Solid Edge part; units mm, degrees
sketch "Sketch1" plane through (0, 0, 0) normal (0, -1, 0) x (1, 0, 0)
  line L0 (0, -16) -> (1.5, -16)
  line L1 (1.5, -16) -> (1.5, -0.601)
  line L2 (1.5, -0.601) -> (1.3375, -0.101)
  line L3 (1.3375, -0.101) -> (1.3375, 0)
  line L4 (1.3375, 0) -> (2.8, 0)
  line L5 (2.8, 0) -> (2.6425, 1.8)
  line L6 (2.6425, 1.8) -> (0, 1.8)
  dimension "D1" = 1.3375
  dimension "D2" = 1.5
  dimension "D3" = 2.6425
revolve "RevolvedProtrusion1" add sketch "Sketch1" angle 360 about axis through (0, 0, 6) along (0, 0, -1)
fillet "Round_1" radius 0.9 1 edges at (-2.6425, 0, 1.8)
sketch "Sketch2" plane through (0, 0, 0) normal (0, -1, 0) x (1, 0, 0)
  line L0 (-0.4, 1.8) -> (-0.4, 1.1)
  line L1 (-0.4, 1.1) -> (0.4, 1.1)
  line L2 (0.4, 1.1) -> (0.4, 1.8)
  line L3 (0.4, 1.8) -> (-0.4, 1.8)
  dimension "D1" = 0.4
  dimension "D2" = 0.4
extrude "ExtrudedCutout_1" cut sketch "Sketch2" along normal mid plane 5.6
cosmetic_thread "Thread_1" thread depth 15.399
fillet "Round_2" radius 0.1 1 edges at (-1.3375, 0, 0)
chamfer "Chamfer_1" distance 0.0012 angle 30 1 edges at (-1.5, 0, -16) measured on face at (1.03, 0.97, -16)
properties material "Steel"
Here's how the part is built. I have some questions about the finished solid (model axes, mm). Coordinates: 2 decimals unless noted, no trailing zeros. Loops run counter-clockwise (first coordinate to the right, second up) from the corner with the lowest first, then second, coordinate; pieces in that order, holes last. Notation, with made-up numbers: M 41,37.25 L 88,37.25 A20 cw 88,74.25 Z; hole C -36,-18.5 d9. An arc over 180 degrees is marked long. One line per item, written item: value.
1. Imagine slicing it at C-C (z = -4.75). List the corners of the cut face in (x, y) for me, and give its area (3 significant figures).
Geometry says:
outline: C 0,0 d3
area: 7.07 mm2
2. Thinking about a two-plate mould opening in X: for faces 1 (the flat face through (0, 0, 1.1)), 2 (the cylindrical face through (-1.5, 0.07, -8.19)), 3 (the flat face through (1.2, 1.2, 0)), which applies, +X half, -X half, draft (parallel to the pull), parting line (faces both ways), or undercut?
Geometry says:
face 1: undercut
face 2: parting line
face 3: draft
3. Will these pins go through, and if not, where does the flat tip stop? pin 1 Ø2 at (x, z) = (-1.5, -7) entering from +Y; pin 2 Ø0.8 at (y, z) = (-1.5, 1.5) entering from -X.
Geometry says:
pin 1: stops at y = 1.41
pin 2: stops at x = -2.37
4. Please list where these lines run through material, in increasing order: probe 1 along Z at (x, y) = (-0.1, -0.75); probe 2 along X at (y, z) = (-2.35, 0.5); probe 3 along Z at (x, y) = (-2.05, 0).
Geometry says:
probe 1: z = -16 to 1.1
probe 2: x = -1.44 to 1.44
probe 3: z = 0 to 1.77
